Build history of the part. All positions in model axes, mm. A direction names the side the tool comes from. Give positions to 0.01 mm unless a question says otherwise; leave off trailing zeros. One line per item, written item: value. Start each with the question number.
from build123d import *

# Parameters (mm, degrees)
F0_W          = 139.7
F0_H          = 139.7
F1_DEPTH      = 2552.7
F2_W          = 38.1
F2_H          = 241.3
F3_DEPTH      = 69.851
F3_DEPTH_BACK = 69.851
F4_W          = 38.1
F4_H          = 241.3
F5_DEPTH      = 69.851
F5_DEPTH_BACK = 69.851
F7_D          = 15.875
F9_D          = 15.875


with BuildPart() as f1:
    # F0 (on Top) → F1 (new body)
    with BuildSketch(Plane.XY):
        Rectangle(F0_W, F0_H)
    extrude(amount=-F1_DEPTH)

    # F2 (on Front) → F3 (cut, two sides)
    with BuildSketch(Plane.XZ) as f3_sk:
        with Locations((50.8, -120.65)):
            Rectangle(F2_W, F2_H)
    extrude(amount=F3_DEPTH, mode=Mode.SUBTRACT)
    extrude(f3_sk.sketch, amount=-F3_DEPTH_BACK, mode=Mode.SUBTRACT)

    # F4 (on Right) → F5 (cut, two sides)
    with BuildSketch(Plane.YZ) as f5_sk:
        with Locations((-50.8, -120.65)):
            Rectangle(F4_W, F4_H)
    extrude(amount=F5_DEPTH, mode=Mode.SUBTRACT)
    extrude(f5_sk.sketch, amount=-F5_DEPTH_BACK, mode=Mode.SUBTRACT)

    # F7 (through all)
    with Locations(Plane.XZ.offset(31.75)):
        with Locations((-19.05, -44.45), (-19.05, -171.45)):
            Hole(F7_D / 2)

    # F9 (through all)
    with Locations(Plane.YZ.offset(31.75)):
        with Locations((19.05, -69.85), (19.05, -196.85)):
            Hole(F9_D / 2)


solid = f1.part
1) Tool access for faces 1 (the face through (-18, -31.75, -122)), 2 (the face through (32, -17, -241.3)), 3 (the face through (31.75, 20, -122)): list every direction of +Z, -Z, +X, -X, +Y, -Y with a clear straight run to the whole face (end or side of a thin tool).
2) Probe line 1 along Z through (x, y) = (1, 19); line 2 along Z through (x, y) = (-19.05, 46.5); line 3 along X through (y, z) = (21, -171). List the from-to ranges inside material, lowest first. Write a range as from..to.
3) Drop flat-ended pins along their axis: P1, Ø20.5, axis at x = -19.05, z = -171.45, coming from the -Y side; P2, Ø9.5, axis at x = -19.05, z = -44.45, coming from the -Y side. Give the stop position or say it passes through.
4) Mould opens along Y. For faces 4 (the face through (-1, -69.85, -1381)), 5 (the face through (-69.85, -1, -1258)), 6 (the face through (-1, 69.85, -1258)) say: released by +Y, released by -Y, zero draft, split by the parting line, or undercut.
Model answer:
1. face 1: +Z, +X, -X, -Y
1. face 2: +Z, +X, -Y
1. face 3: +Z, +X, +Y, -Y
2. line 1: z = -2552.7..-204.79, -188.91..-77.79, -61.91..0
2. line 2: z = -2552.7..-179.39, -163.51..-52.39, -36.51..0
2. line 3: x = -69.85..-26.97, -11.13..31.75
3. P1: stops at y = -31.75
3. P2: passes through
4. face 4: released by -Y
4. face 5: zero draft
4. face 6: released by +Y
